from build123d import *

# Parameters (mm, degrees)
SKETCH1_W               = 127
SKETCH1_H               = 342.9
BOSS_EXTRUDE1_DEPTH     = 12.7
DRAFT1_ANGLE            = -45
CUT_EXTRUDE1_DEPTH      = 184.272045059
CUT_EXTRUDE1_DEPTH_BACK = 5.08
CUT_EXTRUDE2_DEPTH      = 5.08
SKETCH4_W               = 12.7
SKETCH4_H               = 110.871
CUT_EXTRUDE6_DEPTH      = 184.272045059
SKETCH5_W               = 26.162
SKETCH5_H               = 171.958
CUT_EXTRUDE7_DEPTH      = 5.08
FILLET1_R               = 6.604


with BuildPart() as part:
    # Sketch1 → Boss-Extrude1 (new body)
    with BuildSketch(Plane(origin=(0, 0, 0), x_dir=(0, 0, -1), z_dir=(1, 0, 0))):
        Rectangle(SKETCH1_W, SKETCH1_H)
    extrude(amount=BOSS_EXTRUDE1_DEPTH)

    # Draft1
    draft1_faces = [part.faces().sort_by_distance(p)[0] for p in [
        (6.35, -171.45, 0),
        (6.35, 0, -63.5),
        (6.35, 0, 63.5),
        (6.35, 171.45, 0),
    ]]
    draft(draft1_faces, Plane(origin=(0, 0, 0), x_dir=(0, 0, -1), z_dir=(-1, 0, 0)), DRAFT1_ANGLE)

    # Sketch2 → Cut-Extrude1 (cut, two sides: drawn at the far end of the back side and taken through both)
    with BuildSketch(Plane(origin=(12.7, 0, 0), x_dir=(0, 0, -1), z_dir=(1, 0, 0)).offset(-CUT_EXTRUDE1_DEPTH_BACK)):
        with BuildLine():
            Line((-63.5, 19.431), (-30.988, 19.431))
            ThreePointArc((-30.988, 19.431), (-24.384, 12.827), (-30.988, 6.223))
            Line((-30.988, 6.223), (-30.988, -0.508))
            Line((-30.988, -0.508), (63.5, -0.508))
            Line((63.5, -0.508), (63.5, -23.876))
            Line((63.5, -23.876), (-63.5, -23.876))
            Line((-63.5, -23.876), (-63.5, 19.431))
        make_face()
    extrude(amount=CUT_EXTRUDE1_DEPTH + CUT_EXTRUDE1_DEPTH_BACK, mode=Mode.SUBTRACT)

    # Sketch3 → Cut-Extrude2 (cut)
    with BuildSketch(Plane(origin=(12.7, 0, 0), x_dir=(0, 0, -1), z_dir=(1, 0, 0))):
        with BuildLine():
            Line((37.338, -171.45), (63.5, -171.45))
            Line((63.5, -171.45), (63.5, -51.308))
            Line((63.5, -51.308), (46.677466366, -51.308))
            ThreePointArc((46.677466366, -51.308), (37.338, -51.308), (37.338, -60.647466366))
            Line((37.338, -60.647466366), (37.338, -171.45))
        make_face()
    extrude(amount=-CUT_EXTRUDE2_DEPTH, mode=Mode.SUBTRACT)

    # Sketch4 → Cut-Extrude6 (cut, through all)
    with BuildSketch(Plane(origin=(12.7, 0, 0), x_dir=(0, 0, -1), z_dir=(1, 0, 0))):
        with Locations((57.15, -116.0145)):
            Rectangle(SKETCH4_W, SKETCH4_H)
    extrude(amount=-CUT_EXTRUDE6_DEPTH, mode=Mode.SUBTRACT)

    # Sketch5 → Cut-Extrude7 (cut)
    with BuildSketch(Plane(origin=(12.7, 0, 0), x_dir=(0, 0, -1), z_dir=(1, 0, 0))):
        with Locations((50.419, 85.471)):
            Rectangle(SKETCH5_W, SKETCH5_H)
    extrude(amount=-CUT_EXTRUDE7_DEPTH, mode=Mode.SUBTRACT)

    # Fillet1
    fillet1_edges = [part.edges().sort_by_distance(p)[0] for p in [
        (3.81, -60.579, -50.8),
    ]]
    fillet(fillet1_edges, radius=FILLET1_R)


solid = part.part
The listing builds one solid part. Answer for the finished solid, in the listing's coordinates (mm). A direction names the side the tool comes from. Coordinates: 2 decimals unless noted, no trailing zeros. Order: outer loops, then holes, each group sorted by start corner. A loop starts at its lowest first (then second) coordinate and runs counter-clockwise, first axis right, second up. Notation, with made-up numbers: M -33,67 L -9,67 A17 cw -9,72 Z; hole C -39,-11 d2. An arc over 180 degrees is marked long. Use CSV: the item, a comma, the result in double quotes.
Q1. Determine the mould class of faces 4 (the flat face through (7.62, 36, -38)), 5 (the flat face through (3.4, 53.7, -60.1)), 6 (the cylindrical face through (10.2, -51.21, -37.44)), 7 (the flat face through (6.26, 165.19, 0.89)) for opening direction Y: pulls with the +Y half, pulls with the -Y half, needs draft (parallel to the pull), parting line crosses it, or undercut.
Here are the results:
face 4,"undercut"
face 5,"needs draft"
face 6,"undercut"
face 7,"pulls with the +Y half"
Q2. Section A-A (z = 41.5) is taken. Determine the outline of the cut face in (x, y), then the cut area to 3 significant figures.
Here are the results:
outline,"M 0,-171.45 L 12.7,-158.75 L 12.7,-23.88 L 7.62,-23.88 L 7.62,19.43 L 12.7,19.43 L 12.7,158.75 L 0,171.45 Z"
area,"3,970 mm2"
Q3. Section B-B (y = -99) is taken. Determine the outline of the cut face in (x, z), then the cut area to 3 significant figures.
Here are the results:
outline,"M 0,-50.8 L 7.62,-50.8 L 7.62,-37.34 L 12.7,-37.34 L 12.7,50.8 L 0,63.5 Z"
area,"1,300 mm2"
Q4. Given pin 1 Ø4 at (x, y) = (3, -139) entering from -Z; pin 2 Ø2.5 at (x, y) = (9, -88.5) entering from -Z; pin 3 Ø10 at (y, z) = (-97, -43) entering from +X, each flat-ended and moving along its own axis, determine where each tip first touches the part or whether it passes through.
Here are the results:
pin 1,"z = -50.8"
pin 2,"z = -37.34"
pin 3,"x = 7.62"
Q5. Straight lines are drawn through the part: L1, parallel to X at y = -7, z = 46.5; L2, parallel to Y at x = 8.25, z = 9.5; L3, parallel to Y at x = 6, z = 18. For each, find the intervals that lie inside material, in ascending order.
Here are the results:
L1,"0 to 7.62"
L2,"-163.2 to -23.88, -0.51 to 163.2"
L3,"-165.45 to 165.45"
Q6. Section D-D (z = -26.5) is taken. Determine the outline of the cut face in (x, y), then the cut area to 3 significant figures.
Here are the results:
outline,"M 0,-171.45 L 12.7,-158.75 L 12.7,-23.88 L 7.62,-23.88 L 7.62,-0.51 L 12.7,-0.51 L 12.7,158.75 L 0,171.45 Z"
area,"4,070 mm2"
Q7. A tool of negligible diameter and unlimited length cuts with its end or side. For faces 1 (the flat face through (4, -120, -50.8)), 2 (the cylindrical face through (10.124, 12.972, 24.386)), 3 (the flat face through (0, 2, 1)), from which of +Z, -Z, +X, -X, +Y, -Y can it reach the whole face along a straight path? Write none if from no direction.
Here are the results:
face 1,"-Z, +X, -X, -Y"
face 2,"+Z, +X"
face 3,"+Z, -Z, -X, +Y, -Y"
Q8. Section C-C (x = 2.25) is taken. Determine the outline of the cut face in (y, z), then the cut area to 3 significant figures.
Here are the results:
outline,"M -169.2,-50.8 L -67.18,-50.8 A6.6 cw -60.58,-57.4 L -60.58,-61.25 L 169.2,-61.25 L 169.2,61.25 L -169.2,61.25 Z"
area,"40,300 mm2"
